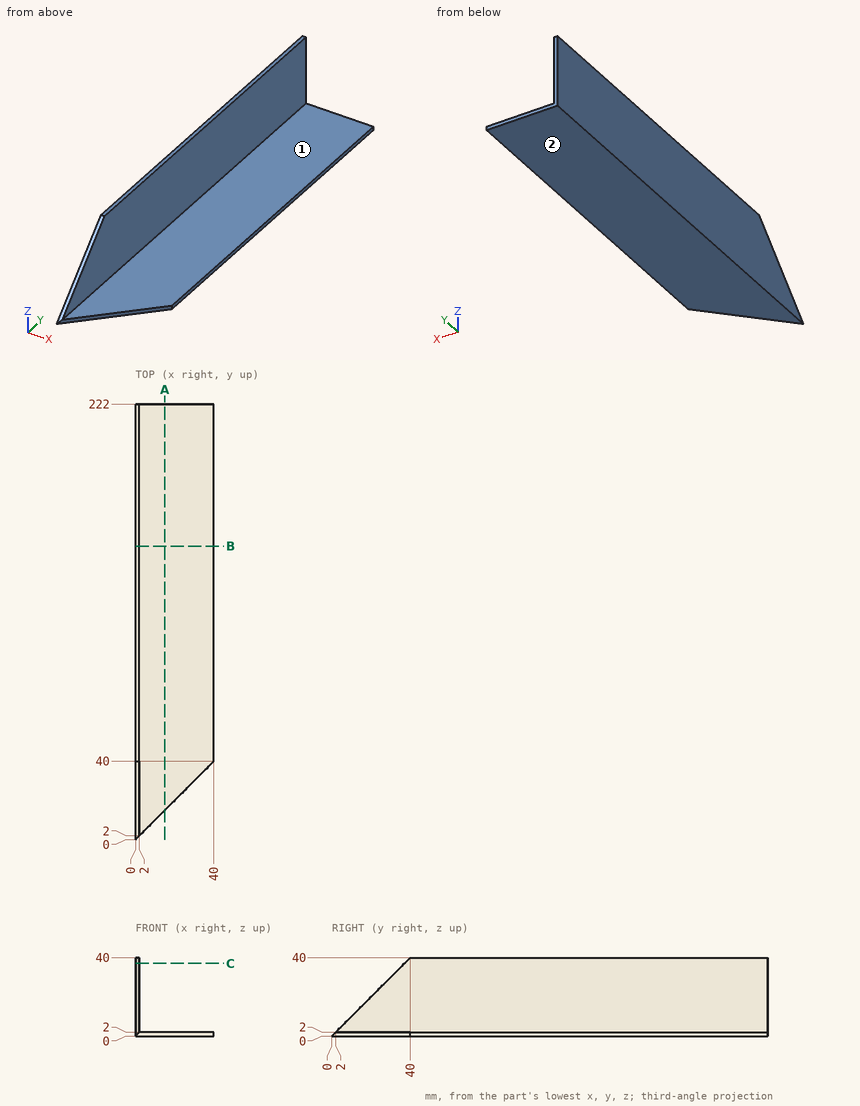
Here's the drawing with two shaded views (mm, measured from the low corner). I have some questions. A direction names the side the tool comes from. Give positions to 0.01 mm unless a question says otherwise; leave off trailing zeros. Write each loop counter-clockwise with the first axis right and the second up, starting at its lowest first coordinate (ties: lowest second). Pieces come first, ordered by that corner, then holes. Notation, with made-up numbers: (39, 43.25) -> (89, 43.25) arc R32 cw to (89, 72.25) -> close; hole circle Ø2 at (-26.75, 65.5). An arc over 180 degrees is marked (long way). Use one line per item in the form item = value. Start each with the question number.
1. Will these pins go through, and if not, where does the flat tip stop? pin 1 Ø2 at (y, z) = (46.5, 11.5) entering from +X; pin 2 Ø10 at (x, y) = (12.5, 183) entering from +Z; pin 3 Ø10 at (x, z) = (35.5, 10) entering from +Y.
2. Imagine slicing it at C-C on z = 37. List the corners of the cut face in (x, y) for me.
3. Imagine slicing it at B-B on y = 149.5. List the corners of the cut face in (x, z) for me, plus the area to 3 significant figures.
4. Imagine slicing it at A-A on x = 15. List the corners of the cut face in (y, z) for me.
5. On a 3-axis mill with a long thin cutter (end or side, diameter ignored), from which of +Z, -Z, +X, -X, +Y, -Y can I reach the whole of each face in a straight line? I mean the marked faces 1 and 2. Say none if no direction works.
6. If I drill on L1, parallel to Z at x = 3.5, y = 64, over which ranges is the centre line in solid material (lowest first)?
Entries:
q1.pin_1 = 2
q1.pin_2 = 2
q1.pin_3 = through
q2.outline = (0, 37) -> (2, 37) -> (2, 222) -> (0, 222) -> close
q3.outline = (0, 0) -> (40, 0) -> (40, 2) -> (2, 2) -> (2, 40) -> (0, 40) -> close
q3.area = 156 mm²
q4.outline = (15, 0) -> (222, 0) -> (222, 2) -> (15, 2) -> close
q5.face_1 = +Z, +X, +Y, -Y
q5.face_2 = -Z, +X, -X, +Y, -Y
q6.L1 = 0 to 2
